from build123d import *

# Parameters (mm, degrees)
SKETCH1_R           = 1
SKETCH1_R_2         = 2
SKETCH1_R_3         = 1.5
BOSS_EXTRUDE1_DEPTH = 2
CHAMFER1_SIZE       = 0.2


with BuildPart() as part:
    # Sketch1 → Boss-Extrude1 (new body)
    with BuildSketch(Plane.XY):
        with BuildLine():
            Line((-18, 3), (18, 3))
            ThreePointArc((18, 3), (21, 0), (18, -3))
            Line((18, -3), (-18, -3))
            ThreePointArc((-18, -3), (-21, 0), (-18, 3))
        make_face()
        with Locations((-18, 0)):
            Circle(SKETCH1_R, mode=Mode.SUBTRACT)
        with Locations((-12, 0)):
            Circle(SKETCH1_R_2, mode=Mode.SUBTRACT)
        with Locations((-4, 0)):
            Circle(SKETCH1_R_2, mode=Mode.SUBTRACT)
        with Locations((18, 0)):
            Circle(SKETCH1_R_3, mode=Mode.SUBTRACT)
        with Locations((12, 0)):
            Circle(SKETCH1_R_2, mode=Mode.SUBTRACT)
        with Locations((4, 0)):
            Circle(SKETCH1_R_2, mode=Mode.SUBTRACT)
    extrude(amount=BOSS_EXTRUDE1_DEPTH)

    # Chamfer1
    chamfer1_edges = [part.edges().sort_by_distance(p)[0] for p in [
        (-19, 0, 0),
        (-19, 0, 2),
        (21, 0, 2),
        (-14, 0, 0),
        (-14, 0, 2),
        (0, 3, 2),
        (-6, 0, 0),
        (-6, 0, 2),
        (16.5, 0, 0),
        (16.5, 0, 2),
        (10, 0, 0),
        (10, 0, 2),
        (2, 0, 0),
        (2, 0, 2),
        (-21, 0, 2),
        (0, 3, 0),
        (21, 0, 0),
        (0, -3, 0),
        (-21, 0, 0),
        (0, -3, 2),
    ]]
    chamfer(chamfer1_edges, length=CHAMFER1_SIZE)


solid = part.part
Design review of the part built by this model. Coordinates are the model's own, in mm. Give positions to 0.01 mm unless a question says otherwise; leave off trailing zeros. Order: outer loops, then holes, each group sorted by start corner. A loop starts at its lowest first (then second) coordinate and runs counter-clockwise, first axis right, second up. Notation, with made-up numbers: (40, 29) - (70, 29) arc R30 cw to (70, 53) - close; hole circle Ø1 at (43, -31). An arc over 180 degrees is marked (long way). Use CSV: the item, a comma, the result in double quotes. Start each with the question number.
Q1. Draft analysis for pull direction Y (two halves, no side actions). For faces 1 (the face through (0, 0, 0)), 2 (the face through (-21, 0, 1)), 3 (the face through (-5.6, -1.2, 1)), 4 (the face through (10.4, -1.2, 1)), state which applies: pulls with the +Y half, pulls with the -Y half, needs draft (parallel to the pull), parting line crosses it, or undercut.
Q2. Take a section at B-B (z = 1.4). State the section outline as (x, y) points, and give its area (3 significant figures).
Q3. For line 1 (X direction, y = 1.7, z = 0.95); line 2 (Y direction, x = 4, z = 0.55); line 3 (X direction, y = -1.1, z = 0.8), list the stretches that pass through material, from the lowest coordinate up.
Q4. Take a section at A-A (x = 12). State the section outline as (y, z) points.
Q5. Take a section at C-C (y = 0). Count the separate pieces of the cut face and the enclosed holes in it, and give its area (3 significant figures).
Q6. For P1, Ø3, axis at x = -4, y = 0, coming from the +Z side, flat-tipped, find the tip position at first contact; note if it passes through.
Calculated:
1,face 1,"needs draft"
1,face 2,"parting line crosses it"
1,face 3,"undercut"
1,face 4,"undercut"
2,outline,"(-18, -3) - (18, -3) arc R3 ccw to (18, 3) - (-18, 3) arc R3 ccw to start; hole circle Ø2 at (-18, 0); hole circle Ø4 at (-12, 0); hole circle Ø4 at (-4, 0); hole circle Ø4 at (4, 0); hole circle Ø4 at (12, 0); hole circle Ø3 at (18, 0)"
2,area,"184 mm²"
3,line 1,"x = -20.47 to -13.05, -10.95 to -5.05, -2.95 to 2.95, 5.05 to 10.95, 13.05 to 20.47"
3,line 2,"y = -3 to -2, 2 to 3"
3,line 3,"x = -20.79 to -13.67, -10.33 to -5.67, -2.33 to 2.33, 5.67 to 10.33, 13.67 to 16.98, 19.02 to 20.79"
4,outline,"(-3, 0.2) - (-2.8, 0) - (-2.2, 0) - (-2, 0.2) - (-2, 1.8) - (-2.2, 2) - (-2.8, 2) - (-3, 1.8) - close; (2, 0.2) - (2.2, 0) - (2.8, 0) - (3, 0.2) - (3, 1.8) - (2.8, 2) - (2.2, 2) - (2, 1.8) - close"
5,separate pieces,"7"
5,enclosed holes,"0"
5,area,"41.4 mm²"
6,P1,"passes through"
